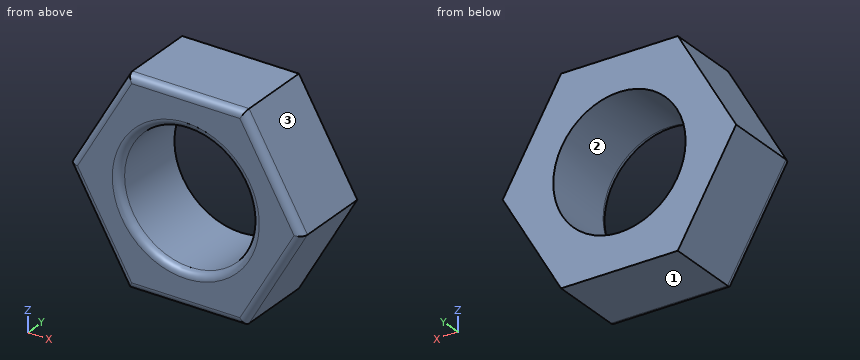
```python
from build123d import *

# Parameters (mm, degrees)
BOSS_EXTRU_1_DEPTH   = 2.2
D_GAGEMENT_M31_D     = 3.6
D_GAGEMENT_M31_DEPTH = 2.2
D_GAGEMENT_M31_TIP   = 1.081549114
CONG_1_R             = 0.2


with BuildPart() as part:
    # Esquisse1 → Boss.-Extru.1 (new body)
    with BuildSketch(Plane(origin=(0, 0, 0), x_dir=(1, 0, 0), z_dir=(0, 1, 0))):
        Polygon((1.58771324, 2.75), (-1.58771324, 2.75), (-3.175426481, 0), (-1.58771324, -2.75), (1.58771324, -2.75), (3.175426481, 0), align=None)
    extrude(amount=BOSS_EXTRU_1_DEPTH)

    # Dégagement M31
    with Locations(Plane(origin=(0, 2.2, 0), x_dir=(1, 0, 0), z_dir=(0, 1, 0))):
        with Locations((0, 0)):
            Hole(D_GAGEMENT_M31_D / 2, depth=D_GAGEMENT_M31_DEPTH)
            with Locations((0, 0, -(D_GAGEMENT_M31_DEPTH + D_GAGEMENT_M31_TIP / 2))):  # 118° drill point
                Cone(0, D_GAGEMENT_M31_D / 2, D_GAGEMENT_M31_TIP, mode=Mode.SUBTRACT)

    # Congé1
    cong_1_edges = [part.edges().sort_by_distance(p)[0] for p in [
        (1.8, 0, 0),
        (2.38156986, 0, 1.375),
        (0, 0, 2.75),
        (-2.38156986, 0, 1.375),
        (-2.38156986, 0, -1.375),
        (0, 0, -2.75),
        (2.38156986, 0, -1.375),
    ]]
    fillet(cong_1_edges, radius=CONG_1_R)


solid = part.part
```
Verification items for the finished model (mm, model axes). Face numbers are marked on the shaded views. Coordinates: 2 decimals unless noted, no trailing zeros. Write each loop counter-clockwise with the first axis right and the second up, starting at its lowest first coordinate (ties: lowest second). Pieces come first, ordered by that corner, then holes. Notation, with made-up numbers: M 45.5,12.5 L 75.5,12.5 A30 ccw 75.5,46.5 Z; hole C 13.25,47 d1. An arc over 180 degrees is marked long. Answer as a JSON object with one key per item and string values. Group by question number.
(1) Material ranges on line 1 (Z direction, x = 0, y = 1.8); line 2 (X direction, y = 0.7, z = -0.65); line 3 (Z direction, x = 0.5, y = 1), recorded low to high.
(2) Release check for a two-part mould opening along Z. For the marked faces 1, 2 and 3 record: +Z half, -Z half, draft (parallel to the pull), parting line (faces both ways), or undercut.
(3) Cross-section at A-A, the plane x = 0. Record the cut outline in (y, z).
(4) Gauge pin test, flat end, axial feed: pin 1 (3 mm diameter, centred on x = 1, z = 0, fed in from -Y). Record the tip position at first contact, or that the pin passes through.
(5) Cross-section at B-B, the plane y = 1.3. Record the cut outline in (x, z).
Reply:
{
 "1": {"line 1": "-2.75 to -1.8, 1.8 to 2.75", "line 2": "-2.8 to -1.68, 1.68 to 2.8", "line 3": "-2.75 to -1.73, 1.73 to 2.75"},
 "2": {"face 1": "-Z half", "face 2": "undercut", "face 3": "+Z half"},
 "3": {"outline": "M 0,-2.55 A0.2 ccw 0.2,-2.75 L 2.2,-2.75 L 2.2,-1.8 L 0.2,-1.8 A0.2 ccw 0,-2 Z; M 0,2 A0.2 ccw 0.2,1.8 L 2.2,1.8 L 2.2,2.75 L 0.2,2.75 A0.2 ccw 0,2.55 Z"},
 "4": {"pin 1": "y = 0"},
 "5": {"outline": "M -3.18,0 L -1.59,-2.75 L 1.59,-2.75 L 3.18,0 L 1.59,2.75 L -1.59,2.75 Z; hole C 0,0 d3.6"}
}
